Verification items for the finished model (mm, model axes). A direction names the side the tool comes from. Round coordinates to 2 decimals unless told otherwise and drop trailing zeros. Write each loop counter-clockwise with the first axis right and the second up, starting at its lowest first coordinate (ties: lowest second). Pieces come first, ordered by that corner, then holes.
from build123d import *

# Parameters (mm, degrees)
SKETCH1_W           = 50
SKETCH1_H           = 45
BODY_DEPTH          = 6
SKETCH4_R           = 16
ROUND_2_DEPTH       = 2
F_1X45_CHAMFER_SIZE = 1
SKETCH5_R           = 3.5
HOLE_1_DEPTH        = 7
HOLES_2_4_COUNT     = 4
R4_FILLETS_R        = 4
R1_FILLET_R         = 1


with BuildPart() as part:
    # Sketch1 → Body (new body)
    with BuildSketch(Plane(origin=(0, 0, 0), x_dir=(1, 0, 0), z_dir=(0, 1, 0))):
        with Locations((3, 0)):
            Rectangle(SKETCH1_W, SKETCH1_H)
    extrude(amount=BODY_DEPTH)

    # Sketch4 → Round 2 (add)
    with BuildSketch(Plane.XZ):
        Circle(SKETCH4_R)
    extrude(amount=ROUND_2_DEPTH)

    # 1x45 Chamfer
    f_1x45_chamfer_edges = [part.edges().sort_by_distance(p)[0] for p in [
        (-16, -2, 0),
    ]]
    chamfer(f_1x45_chamfer_edges, length=F_1X45_CHAMFER_SIZE)

    # Sketch5 → Hole 1 (cut, through all)
    with BuildSketch(Plane.XZ):
        with Locations((16.263455967, 16.263455967)):
            Circle(SKETCH5_R)
    hole_1 = extrude(amount=-HOLE_1_DEPTH, mode=Mode.SUBTRACT)

    # Holes 2-4: Hole 1 ×4 about axis
    holes_2_4_axis = Axis((0, 0, 0), (0, 1, 0))
    for i in range(1, HOLES_2_4_COUNT):
        add(hole_1.rotate(holes_2_4_axis, i * 360 / HOLES_2_4_COUNT), mode=Mode.SUBTRACT)

    # R4 Fillets
    r4_fillets_edges = [part.edges().sort_by_distance(p)[0] for p in [
        (-22, 3, -22.5),
        (28, 3, -22.5),
        (28, 3, 22.5),
        (-22, 3, 22.5),
    ]]
    fillet(r4_fillets_edges, radius=R4_FILLETS_R)

    # R1 Fillet
    r1_fillet_edges = [part.edges().sort_by_distance(p)[0] for p in [
        (-22, 6, 0),
        (3, 6, -22.5),
        (3, 6, 22.5),
        (28, 6, 0),
        (26.828427125, 6, 21.328427125),
        (-20.828427125, 6, 21.328427125),
        (26.828427125, 6, -21.328427125),
        (-20.828427125, 6, -21.328427125),
    ]]
    fillet(r1_fillet_edges, radius=R1_FILLET_R)


solid = part.part
Q1. Tool access check on faces 1 (the flat face through (3, 2, 22.5)), 2 (the cylindrical face through (-3.47, -0.49, -15.62)). Record the directions out of +Z, -Z, +X, -X, +Y, -Y that give a thin tool (end or side, any length) a straight path to the whole face; none if there is none.
Recorded:
face 1: +Z, +X, -X, +Y, -Y
face 2: -Y
Q2. Sectioned sample at B-B (x = 0). Enter the section's corners in (y, z).
Recorded:
outline: (-2, -15) - (-1, -16) - (0, -16) - (0, -22.5) - (5, -22.5) arc R1 ccw to (6, -21.5) - (6, 21.5) arc R1 ccw to (5, 22.5) - (0, 22.5) - (0, 16) - (-1, 16) - (-2, 15) - close
Q3. Release check for a two-part mould opening along Z. For faces 3 (the cylindrical face through (-20.859, 2.535, -21.297)), 4 (the cylindrical face through (-13.16, 2.96, 17.88)), 5 (the flat face through (-22, 2, 0)) record: released by +Z, released by -Z, zero draft, split by the parting line, or undercut.
Recorded:
face 3: released by -Z
face 4: undercut
face 5: zero draft
Q4. Depth check by flat-ended pin: P1, Ø8, axis at x = 16.26, z = 16.26, coming from the -Y side. Enter the tip coordinate at first touch or a pass-through.
Recorded:
P1: stops at y = 0
Q5. Sectioned sample at C-C (y = 1.25). Enter the section's corners in (x, z), plus the area to 3 significant figures.
Recorded:
outline: (-22, -18.5) arc R4 ccw to (-18, -22.5) - (24, -22.5) arc R4 ccw to (28, -18.5) - (28, 18.5) arc R4 ccw to (24, 22.5) - (-18, 22.5) arc R4 ccw to (-22, 18.5) - close; hole circle Ø7 at (-16.26, -16.26); hole circle Ø7 at (-16.26, 16.26); hole circle Ø7 at (16.26, -16.26); hole circle Ø7 at (16.26, 16.26)
area: 2,080 mm2
Q6. Material ranges on line 1 along X through (y, z) = (3.5, -15.5); line 2 along X through (y, z) = (1.5, 19); line 3 along Z through (x, y) = (-14.5, 1.25), recorded low to high.
Recorded:
line 1: x = -22 to -19.68, -12.85 to 12.85, 19.68 to 28
line 2: x = -21.97 to -18.45, -14.08 to 14.08, 18.45 to 27.97
line 3: z = -22.5 to -19.29, -13.24 to 13.24, 19.29 to 22.5
Q7. Sectioned sample at D-D (x = 13.5). Give the number of separate pieces and of enclosed holes in the cut face, plus the area to 3 significant figures.
Recorded:
separate pieces: 3
enclosed holes: 0
area: 250 mm2
Q8. Sectioned sample at A-A (z = 0). Enter the section's corners in (x, y).
Recorded:
outline: (-22, 0) - (-16, 0) - (-16, -1) - (-15, -2) - (15, -2) - (16, -1) - (16, 0) - (28, 0) - (28, 5) arc R1 ccw to (27, 6) - (-21, 6) arc R1 ccw to (-22, 5) - close
